Can you work these out from the model? Positions are in its coordinate system, mm. A direction names the side the tool comes from. Coordinates: 2 decimals unless noted, no trailing zeros. Write each loop counter-clockwise with the first axis right and the second up, starting at its lowest first coordinate (ties: lowest second). Pieces come first, ordered by that corner, then holes. Notation, with made-up numbers: (47, 46) - (71, 46) arc R14 ccw to (71, 70) - close; hole circle Ø8 at (49.5, 82). An arc over 180 degrees is marked (long way). Use one line per item in the form item = value. Start each with the question number.
(1) If we section it at C-C on z = 3.35: Please give me the cut outline in (x, y), then the cut area to 3 significant figures.
(2) If I drill on probe 1 along Y at (x, z) = (-0.5, 1.9); probe 2 along X at (y, z) = (-13, 1); probe 3 along X at (y, z) = (-16, 0.4), over which ranges is the centre line in solid material (lowest first)? Write a range as from..to.
(3) On a 3-axis mill with a long thin cutter (end or side, diameter ignored), from which of +Z, -Z, +X, -X, +Y, -Y can I reach the whole of each face in a straight line? I mean faces 1 (the face through (16, -39, 1)), 2 (the face through (-6.3, -22.2, 1.5)), 3 (the face through (36.843, -23, 1)). Say none if no direction works.
(4) Thinking about a two-plate mould opening in Y: for faces 4 (the face through (-3.461, -23, 1)), 5 (the face through (15, -45, 1)), 6 (the face through (39.5, -22.82, 0.57)), which applies, pulls with the +Y half, pulls with the -Y half, needs draft (parallel to the pull), parting line crosses it, or undercut?
(5) If we section it at A-A on y = -38: Please give me the cut outline in (x, z), then the cut area to 3 significant figures.
(6) For pin 1 Ø4 at (x, y) = (-8.5, -11.5) entering from +Z; pin 2 Ø1 at (x, y) = (-3.5, -6) entering from +Z; pin 3 Ø0.6 at (y, z) = (-23.5, 1.5) entering from -X, each with a flat end and sliding along its axis, tell me the tip position at first contact or that it passes through.
(7) If we section it at B-B on x = 23: Please give me the cut outline in (y, z).
```python
from build123d import *

# Parameters (mm, degrees)
F1_DEPTH = 45
F2_R     = 2
F3_W     = 40.303819
F3_H     = 33
F4_DEPTH = 2.1


with BuildPart() as f1:
    # F0 (on Front) → F1 (new body)
    with BuildSketch(Plane.XZ):
        Polygon((-6.300002, 0.9), (-9.900002, 0.9), (-9.900002, 0), (40.099998, 0), (40.099998, 2.1), (37.999998, 2.1), (-6.300002, 2.1), align=None)
        Polygon((37.999998, 2.1), (40.099998, 2.1), (40.099998, 4.2), (36.499998, 4.2), align=None)
    extrude(amount=F1_DEPTH)

    # F2
    f2_edges = [f1.edges().sort_by_distance(p)[0] for p in [
        (40.099998, -22.5, 4.2),
        (40.099998, -22.5, 0),
    ]]
    fillet(f2_edges, radius=F2_R)

    # F3 (on face) → F4 (cut)
    with BuildSketch(Plane.XY.offset(2.1)):
        with Locations((16.690705, -22.5)):
            Rectangle(F3_W, F3_H)
    extrude(amount=-F4_DEPTH, mode=Mode.SUBTRACT)


solid = f1.part
```
Reported:
q1.outline = (37.11, -45) - (39.74, -45) - (39.74, 0) - (37.11, 0) - close
q1.area = 118 mm2
q2.probe_1 = -45..-39, -6..0
q2.probe_2 = -6.3..-3.46, 36.84..39.83
q2.probe_3 = -9.9..-3.46, 36.84..39.3
q3.face_1 = +Z, -Z
q3.face_2 = +Z, -X, +Y, -Y
q3.face_3 = -Z
q4.face_4 = undercut
q4.face_5 = pulls with the -Y half
q4.face_6 = needs draft
q5.outline = (-9.9, 0) - (-3.46, 0) - (-3.46, 2.1) - (-6.3, 2.1) - (-6.3, 0.9) - (-9.9, 0.9) - close; (36.5, 4.2) - (38, 2.1) - (36.84, 2.1) - (36.84, 0) - (38.1, 0) arc R2 ccw to (40.1, 2) - (40.1, 2.2) arc R2 ccw to (38.1, 4.2) - close
q5.area = 20.3 mm2
q6.pin_1 = 0.9
q6.pin_2 = 2.1
q6.pin_3 = -6.3
q7.outline = (-45, 0) - (-39, 0) - (-39, 2.1) - (-45, 2.1) - close; (-6, 0) - (0, 0) - (0, 2.1) - (-6, 2.1) - close
